Design review of the part built by this model. Coordinates are the model's own, in mm. Face numbers are marked on the shaded views. A direction names the side the tool comes from. Coordinates: 2 decimals unless noted, no trailing zeros. Loops run counter-clockwise (first coordinate to the right, second up) from the corner with the lowest first, then second, coordinate; pieces in that order, holes last. Notation, with made-up numbers: (64.25, 58.25) - (103.25, 58.25) arc R29 ccw to (103.25, 80.25) - close; hole circle Ø6 at (72, -32). An arc over 180 degrees is marked (long way). Use one line per item in the form item = value. Start each with the question number.
(1) Add section D-D (x = 29). State the section outline as (y, z) points.
(2) Add section B-B (y = 24.5). State the section outline as (x, z) points, plus the area to 3 significant figures.
(3) The part is to be moulded in two halves that separate along Z. For the marked faces 6, 7, 8 and 9, say which applies: pulls with the +Z half, pulls with the -Z half, needs draft (parallel to the pull), parting line crosses it, or undercut.
(4) For L1, parallel to Y at x = 50.5, z = -13; L2, parallel to X at y = 18.5, z = -37; L3, parallel to X at y = 38, z = -55.5, list the stretches that pass through material, from the lowest coordinate up.
(5) Add section C-C (z = -57). State the section outline as (x, y) points.
(6) Tool access review of the marked faces 1, 2, 3, 4 and 5: name each direction out of +Z, -Z, +X, -X, +Y, -Y from which nothing blocks a thin tool from reaching the whole face with its end or side.
(7) Clearance check with flat-ended pins moving along their axes: pin 1 Ø18.5 at (x, y) = (29.5, 81.5) entering from -Z; pin 2 Ø3 at (x, y) = (59, 58.5) entering from +Z; pin 3 Ø20.5 at (y, z) = (103.5, -29) entering from +X. State where each tip first meets the part, or that it passes through.
(8) Add section A-A (z = -9). State the section outline as (x, y) points.
```python
from build123d import *

# Parameters (mm, degrees)
SKETCH1_W               = 70
SKETCH1_H               = 65
BOSS_EXTRUDE1_DEPTH     = 20
SKETCH2_W               = 45
SKETCH2_H               = 35
CUT_EXTRUDE1_DEPTH      = 10
SKETCH3_W               = 70
SKETCH3_H               = 17.205499322
BOSS_EXTRUDE2_DEPTH     = 75
CUT_EXTRUDE2_REACH      = 136.722
CUT_EXTRUDE3_REACH      = 136.722
CUT_EXTRUDE3_END_RADIUS = 29.761393769
SKETCH7_W               = 28.5
SKETCH7_H               = 6.302488938
SKETCH8_W               = 70
SKETCH8_H               = 17.205499322
BOSS_EXTRUDE3_DEPTH     = 15
CUT_EXTRUDE4_DEPTH      = 146.688022843
CUT_EXTRUDE4_DEPTH_BACK = 146.688022843
BOSS_EXTRUDE8_START     = 40.5
BOSS_EXTRUDE8_DEPTH     = 40.5
BOSS_EXTRUDE10_DEPTH    = 40.5


with BuildPart() as part:
    # Sketch1 → Boss-Extrude1 (new body)
    with BuildSketch(Plane(origin=(0, 0, 0), x_dir=(1, 0, 0), z_dir=(0, 1, 0))):
        with Locations((35, 32.5)):
            Rectangle(SKETCH1_W, SKETCH1_H)
    extrude(amount=BOSS_EXTRUDE1_DEPTH)

    # Sketch2 → Cut-Extrude1 (cut)
    with BuildSketch(Plane(origin=(0, 20, 0), x_dir=(1, 0, 0), z_dir=(0, 1, 0))):
        with Locations((35.6, 25.150369075)):
            Rectangle(SKETCH2_W, SKETCH2_H)
    extrude(amount=-CUT_EXTRUDE1_DEPTH, mode=Mode.SUBTRACT)

    # Sketch3 → Boss-Extrude2 (add)
    with BuildSketch(Plane(origin=(0, 20, 0), x_dir=(1, 0, 0), z_dir=(0, 1, 0))):
        with Locations((35, 56.397250339)):
            Rectangle(SKETCH3_W, SKETCH3_H)
    extrude(amount=BOSS_EXTRUDE2_DEPTH)

    # Sketch6 → Cut-Extrude2 (cut, up to next)
    with BuildSketch(Plane(origin=(0, 0, -65), x_dir=(-1, 0, 0), z_dir=(0, 0, -1)), mode=Mode.PRIVATE) as cut_extrude2_sk1:
        with BuildLine():
            Line((-61, 60), (-61, 20))
            Line((-61, 20), (-9, 20))
            Line((-9, 20), (-9, 60))
            ThreePointArc((-9, 60), (-35, 75.278971352), (-61, 60))
        make_face()
    cut_extrude2_tool1 = extrude(cut_extrude2_sk1.sketch, amount=-CUT_EXTRUDE2_REACH, mode=Mode.PRIVATE) & part.part
    add(cut_extrude2_tool1.solids().sort_by_distance((35, 45.608619, -65))[0], mode=Mode.SUBTRACT)

    # Cut-Extrude3: up to this cylinder (the profile starts outside it)
    cut_extrude3_end = Plane(origin=(35, 45.517577583, -61.848756), z_dir=(0, 0, -1)) * Cylinder(CUT_EXTRUDE3_END_RADIUS, 333.966787538, mode=Mode.PRIVATE)
    # Sketch7 → Cut-Extrude3 (cut, up to the surface)
    with BuildSketch(Plane(origin=(0, 95, 0), x_dir=(1, 0, 0), z_dir=(0, 1, 0)), mode=Mode.PRIVATE) as cut_extrude3_sk1:
        with Locations((35, 61.848755531)):
            Rectangle(SKETCH7_W, SKETCH7_H)
    cut_extrude3_tool1 = extrude(cut_extrude3_sk1.sketch, amount=-CUT_EXTRUDE3_REACH, mode=Mode.PRIVATE) - cut_extrude3_end
    add(cut_extrude3_tool1.solids().sort_by_distance((35, 95, -61.848756))[0], mode=Mode.SUBTRACT)

    # Sketch8 → Boss-Extrude3 (add)
    with BuildSketch(Plane(origin=(0, 95, 0), x_dir=(1, 0, 0), z_dir=(0, 1, 0))):
        with Locations((35, 56.397250339)):
            Rectangle(SKETCH8_W, SKETCH8_H)
    extrude(amount=BOSS_EXTRUDE3_DEPTH)

    # Sketch9 → Cut-Extrude4 (cut, two sides: drawn at the far end of the back side and taken through both)
    with BuildSketch(Plane(origin=(0, 0, -65), x_dir=(-1, 0, 0), z_dir=(0, 0, -1)).offset(-CUT_EXTRUDE4_DEPTH_BACK)):
        with BuildLine():
            Line((-168.040562266, 331.160425887), (-49.25, 110))
            ThreePointArc((-49.25, 110), (-35, 101.478526665), (-20.75, 110))
            Line((-20.75, 110), (98.040562266, 331.160425887))
            Line((98.040562266, 331.160425887), (98.040562266, 833.248592098))
            Line((98.040562266, 833.248592098), (-168.040562266, 833.248592098))
            Line((-168.040562266, 833.248592098), (-168.040562266, 331.160425887))
        make_face()
    extrude(amount=CUT_EXTRUDE4_DEPTH + CUT_EXTRUDE4_DEPTH_BACK, mode=Mode.SUBTRACT)

    # Sketch10 → Boss-Extrude8 (add)
    with BuildSketch(Plane.XY.offset(-47.794500678).offset(BOSS_EXTRUDE8_START)):
        with BuildLine():
            Line((49.25, 110), (55.25, 110))
            Line((55.25, 110), (55.25, 97.797353367))
            Line((55.25, 97.797353367), (20.533128671, 97.797353367))
            Line((20.533128671, 97.797353367), (14.75, 97.797353367))
            Line((14.75, 97.797353367), (14.75, 110))
            Line((14.75, 110), (20.75, 110))
            ThreePointArc((20.75, 110), (35, 101.478526665), (49.25, 110))
        make_face()
    extrude(amount=-BOSS_EXTRUDE8_DEPTH)

    # Sketch12 → Boss-Extrude10 (add)
    with BuildSketch(Plane.ZY.offset(-14.75)):
        with BuildLine():
            Line((-16.303904233, 97.797353367), (-47.794500678, 97.797353367))
            Line((-47.794500678, 97.797353367), (-47.794500678, 84.67575775))
            ThreePointArc((-47.794500678, 84.67575775), (-33.03291757, 93.597379394), (-16.303904233, 97.797353367))
        make_face()
    extrude(amount=-BOSS_EXTRUDE10_DEPTH)


solid = part.part
```
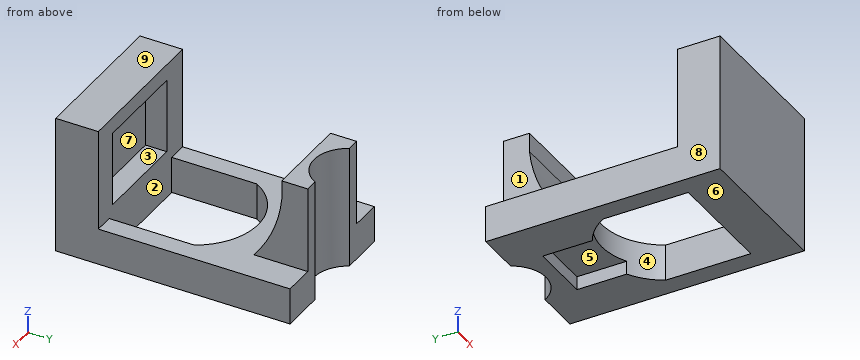
Computed values:
q1.outline = (0, -65) - (20, -65) - (20, -42.65) - (10, -42.65) - (10, -7.65) - (20, -7.65) - (20, 0) - (0, 0) - close; (74.67, -58.7) - (95, -58.7) - (95, -65) - (102.63, -65) - (102.63, -7.29) - (97.8, -7.29) - (97.8, -16.3) arc R58.16 cw to (84.68, -47.79) - (74.67, -47.79) - close
q2.outline = (0, -65) - (9, -65) - (9, -47.79) - (0, -47.79) - close; (61, -65) - (70, -65) - (70, -47.79) - (61, -47.79) - close
q2.area = 310 mm^2
q3.face_6 = pulls with the -Z half
q3.face_7 = undercut
q3.face_8 = needs draft
q3.face_9 = pulls with the +Z half
q4.L1 = 0 to 10, 97.8 to 110
q4.L2 = 0 to 13.1, 58.1 to 70
q4.L3 = 0 to 9, 61 to 70
q5.outline = (0, 0) - (70, 0) - (70, 110) - (49.25, 110) arc R16.18 cw to (20.75, 110) - (0, 110) - close; hole (9, 20) - (61, 20) - (61, 60) arc R29.76 ccw to (9, 60) - close
q6.face_1 = +Z, -X, +Y
q6.face_2 = +Z
q6.face_3 = none
q6.face_4 = +Z, -Z
q6.face_5 = -Z
q7.pin_1 = -65
q7.pin_2 = through
q7.pin_3 = 55.25
q8.outline = (0, 0) - (70, 0) - (70, 20) - (58.1, 20) - (58.1, 10) - (13.1, 10) - (13.1, 20) - (0, 20) - close; (14.75, 97.8) - (55.25, 97.8) - (55.25, 110) - (49.25, 110) arc R16.18 cw to (20.75, 110) - (14.75, 110) - close
